```python
from build123d import *

# Parameters (mm, degrees)
F0_R     = 2.5
F1_DEPTH = 15
F0_R_2   = 6.3158003242
F2_DEPTH = 1.5


# Not quite as in the source:
# - a fillet or chamfer that OpenCascade refuses, or shapes differently, is made with other operations: its cross-section is extruded or revolved along the edge and cut away or added


with BuildPart() as f1:
    # F0 (on Front) → F1 (new body)
    with BuildSketch(Plane.XZ):
        Circle(F0_R)
    extrude(amount=F1_DEPTH)

    # F0 (on Front) → F2 (join)
    with BuildSketch(Plane.XZ):
        Circle(F0_R_2)
        Circle(F0_R, mode=Mode.SUBTRACT)
    extrude(amount=F2_DEPTH)

    # F3: fillet of radius 2 on 1 edges, made by hand

    # F3_s1 → F3_t2 (revolve, cut)
    with BuildSketch(Plane.XY):
        with BuildLine():
            ThreePointArc((6.3158003242, -1.5), (5.6040535225, -0.4188611699), (4.3793086511, 0))
            Line((4.3793086511, 0), (6.3158003242, 0))
            Line((6.3158003242, 0), (6.3158003242, -1.5))
        make_face()
    revolve(axis=Axis((0, 0, 0), (0, -1, 0)), mode=Mode.SUBTRACT)


solid = f1.part
```
Geometry: final body of the model. Coordinates: model frame, mm. A direction names the side the tool comes from. Give positions to 0.01 mm unless a question says otherwise; leave off trailing zeros. Order: outer loops, then holes, each group sorted by start corner. A loop starts at its lowest first (then second) coordinate and runs counter-clockwise, first axis right, second up. Notation, with made-up numbers: (73, 26.25) -> (126, 26.25) arc R11 ccw to (126, 39.25) -> close; hole circle Ø6 at (21.5, 52). An arc over 180 degrees is marked (long way). Write each question's results on one line, items separated by ' | '. Start each with the question number.
1) First-contact query: pin 1 (2 mm diameter, centred on x = 3, z = 2.5, fed in from -Y); pin 2 (6 mm diameter, centred on x = 4.5, y = -11.5, fed in from -Z); pin 3 (3 mm diameter, centred on x = 2.5, y = -11, fed in from -Z). Flat tips, straight axial feed; report the tip coordinate or a pass-through.
2) Section A-A (z = 0). Return loops of the section in (x, y), then the cut area to 3 significant figures.
3) Line query: line 1 (Y direction, x = 2.5, z = -2.75); line 2 (Z direction, x = -1.25, y = -14.25); line 3 (X direction, y = -4.75, z = -0.5). Output: solid intervals per line, ascending. Write a range as from..to.
4) Section B-B (x = 0). Return loops of the section in (y, z), then the cut area to 3 significant figures.
5) Section C-C (y = -8.25). Return loops of the section in (x, z), then the cut area to 3 significant figures.
6) Set-up query: faces 1 (the cylindrical face through (-0.54, -8.16, -2.44)), 2 (the flat face through (0, -15, 0)). Return all of +Z, -Z, +X, -X, +Y, -Y with unobstructed straight access to the full face (end or side cutting, diameter ignored); none if empty.
Calculated:
1) pin 1: y = -1.5 | pin 2: z = -2 | pin 3: z = -2.29
2) outline: (-6.32, -1.5) -> (-2.5, -1.5) -> (-2.5, -15) -> (2.5, -15) -> (2.5, -1.5) -> (6.32, -1.5) arc R2 ccw to (4.38, 0) -> (-4.38, 0) arc R2 ccw to start | area: 84.9 mm2
3) line 1: -1.5..0 | line 2: -2.17..2.17 | line 3: -2.45..2.45
4) outline: (-15, -2.5) -> (-1.5, -2.5) -> (-1.5, -6.32) arc R2 ccw to (0, -4.38) -> (0, 4.38) arc R2 ccw to (-1.5, 6.32) -> (-1.5, 2.5) -> (-15, 2.5) -> close | area: 84.9 mm2
5) outline: circle Ø5 at (0, 0) | area: 19.6 mm2
6) face 1: -Y | face 2: +Z, -Z, +X, -X, -Y
